For this review, take the finished solid that the model builds, in its own axes (mm). A direction names the side the tool comes from. Coordinates: 2 decimals unless noted, no trailing zeros. Loops run counter-clockwise (first coordinate to the right, second up) from the corner with the lowest first, then second, coordinate; pieces in that order, holes last. Notation, with made-up numbers: M 88.25,-18.5 L 113.25,-18.5 A12 cw 113.25,1.5 Z; hole C 31,30 d4. An arc over 180 degrees is marked long. Write each question's results on one line, items separated by ' | '. Start each with the question number.
```python
from build123d import *

# Parameters (mm, degrees)
F0_W     = 6.5
F0_H     = 6.5
F1_DEPTH = 42
F3_DEPTH = 29.801


with BuildPart() as f1:
    # F0 (on Top) → F1 (new body)
    with BuildSketch(Plane.XY):
        Polygon((20.5, 0), (0, 0), (0, -29.8), (10.5, -29.8), (10.5, -2), (20.5, -2), align=None)
        with Locations((5.25, -24.55)):
            Rectangle(F0_W, F0_H, mode=Mode.SUBTRACT)
        with Locations((5.25, -5.25)):
            Rectangle(F0_W, F0_H, mode=Mode.SUBTRACT)
    extrude(amount=F1_DEPTH)

    # F2 (on face) → F3 (cut, through all)
    with BuildSketch(Plane(origin=(0, 0, 0), x_dir=(-1, 0, 0), z_dir=(0, 1, 0))):
        with BuildLine():
            Line((-15.9, 5.5), (-14.15, 5.5))
            ThreePointArc((-14.15, 5.5), (-14.6625631329, 6.7374368671), (-15.9, 7.25))
            Line((-15.9, 7.25), (-15.9, 5.5))
        make_face()
        with BuildLine():
            Line((-15.9, 5.5), (-15.9, 3.75))
            ThreePointArc((-15.9, 3.75), (-14.6625631329, 4.2625631329), (-14.15, 5.5))
            Line((-14.15, 5.5), (-15.9, 5.5))
        make_face()
        with BuildLine():
            ThreePointArc((-15.9, 7.25), (-17.65, 5.5), (-15.9, 3.75))
            Line((-15.9, 3.75), (-15.9, 5.5))
            Line((-15.9, 5.5), (-15.9, 7.25))
        make_face()
        with BuildLine():
            ThreePointArc((-15.9, 35.25), (-14.6625631329, 35.7625631329), (-14.15, 37))
            Line((-14.15, 37), (-15.9, 37))
            Line((-15.9, 37), (-15.9, 35.25))
        make_face()
        with BuildLine():
            Line((-15.9, 37), (-14.15, 37))
            ThreePointArc((-14.15, 37), (-17.1374368671, 38.2374368671), (-15.9, 35.25))
            Line((-15.9, 35.25), (-15.9, 37))
        make_face()
    extrude(amount=-F3_DEPTH, mode=Mode.SUBTRACT)


solid = f1.part
```
Q1. Take a section at D-D, the plane x = 16.75. Give the boundary of the cut face in (y, z), then the cut area to 3 significant figures.
Q2. Take a section at A-A, the plane z = 11. Give the boundary of the cut face in (x, y), then the cut area to 3 significant figures.
Q3. The part is to be moulded in two halves that separate along X. For faces 4 (the face through (5, -29.8, 21)), 5 (the face through (10.5, -16, 21)), 6 (the face through (5, -21.3, 21)), say which applies: pulls with the +X half, pulls with the -X half, needs draft (parallel to the pull), parting line crosses it, or undercut.
Q4. To check wall thickness, follow line 1 along Z through (x, y) = (15.9, -0.9); line 2 along Y through (x, z) = (5, 39.5); line 3 along X through (y, z) = (-0.95, 37). State the ranges of each line that lie inside material, in increasing order.
Q5. Insertion check: P1, Ø4.5, axis at x = 15.9, z = 37, coming from the -Y side; P2, Ø4, axis at y = -17.5, z = 6.5, coming from the +X side. Each pin has a flat end and moves straight along its axis. Give the tip position at first contact, or say it passes through.
Q6. Take a section at B-B, the plane y = -23.5. Give the boundary of the cut face in (x, z).
Q7. For faces 1 (the face through (15, -2, 21)), 2 (the face through (10, 0, 21)), 3 (the face through (5, -2, 21)), list the 3-axis set-ups (+Z, -Z, +X, -X, +Y, -Y) from which the entire face can be reached by the end or side of a thin tool; tool diameter is ignored.
Q8. Take a section at C-C, the plane x = 8. Give the boundary of the cut face in (y, z), then the cut area to 3 significant figures.
Results:
1) outline: M -2,0 L 0,0 L 0,3.97 L -2,3.97 Z; M -2,7.03 L 0,7.03 L 0,35.47 L -2,35.47 Z; M -2,38.53 L 0,38.53 L 0,42 L -2,42 Z | area: 71.8 mm^2
2) outline: M 0,-29.8 L 10.5,-29.8 L 10.5,-2 L 20.5,-2 L 20.5,0 L 0,0 Z; hole M 2,-27.8 L 8.5,-27.8 L 8.5,-21.3 L 2,-21.3 Z; hole M 2,-8.5 L 8.5,-8.5 L 8.5,-2 L 2,-2 Z | area: 248 mm^2
3) face 4: needs draft | face 5: pulls with the +X half | face 6: undercut
4) line 1: 0 to 3.75, 7.25 to 35.25, 38.75 to 42 | line 2: -29.8 to -27.8, -21.3 to -8.5, -2 to 0 | line 3: 0 to 14.15, 17.65 to 20.5
5) P1: y = -2 | P2: x = 10.5
6) outline: M 0,0 L 2,0 L 2,42 L 0,42 Z; M 8.5,0 L 10.5,0 L 10.5,42 L 8.5,42 Z
7) face 1: +Z, -Z, +X, -Y | face 2: +Z, -Z, +X, -X, +Y | face 3: +Z, -Z
8) outline: M -29.8,0 L -27.8,0 L -27.8,42 L -29.8,42 Z; M -21.3,0 L -8.5,0 L -8.5,42 L -21.3,42 Z; M -2,0 L 0,0 L 0,42 L -2,42 Z | area: 706 mm^2
